Verification items for the finished model (mm, model axes). Round coordinates to 2 decimals unless told otherwise and drop trailing zeros. Write each loop counter-clockwise with the first axis right and the second up, starting at its lowest first coordinate (ties: lowest second). Pieces come first, ordered by that corner, then holes. Notation, with made-up numbers: M 47.25,28.5 L 78.25,28.5 A13 ccw 78.25,36.5 Z; hole C -5,89.25 d2. An arc over 180 degrees is marked long. One line per item, written item: value. Start each with the question number.
Item 1: Section check A-A, the plane x = -90.5. Record the cut outline in (y, z) (3 decimals).
Item 2: Section check C-C, the plane x = -71. Record the cut outline in (y, z) (1 decimal).
Item 3: Thickness scan on probe 1 along X at (y, z) = (-37.5, 1.1); probe 2 along X at (y, z) = (-17, 0.45); probe 3 along Y at (x, z) = (-71.5, 3). Record the ranges inside material, lowest first. Write a range as from..to.
Item 4: Gauge pin test, flat end, axial feed: pin 1 (18.5 mm diameter, centred on x = -76.93, y = -28.23, fed in from -Z). Record the tip position at first contact, or that the pin passes through.
Item 5: Section check D-D, the plane y = -11.5. Record the cut outline in (x, z) (3 decimals), then the cut area to 3 significant figures.
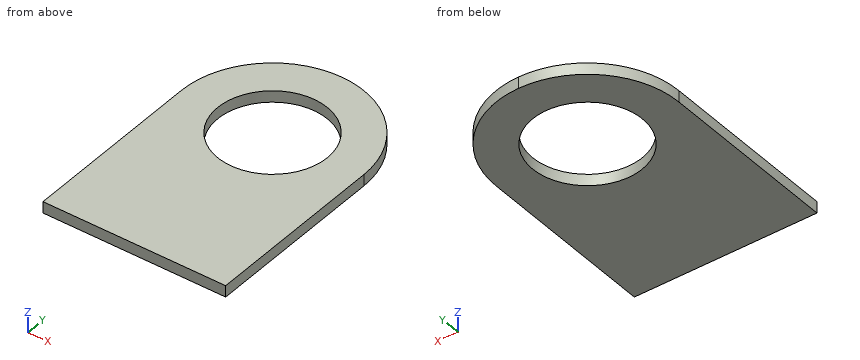
from build123d import *

# Parameters (mm, degrees)
SKETCH1_W           = 50.8
SKETCH1_H           = 76.2
SKETCH1_R           = 15.24
BOSS_EXTRUDE1_DEPTH = 3.175
FILLET1_R           = 25.4


with BuildPart() as part:
    # Sketch1 → Boss-Extrude1 (new body)
    with BuildSketch(Plane.XY):
        with Locations((-76.925714286, -40.930285714)):
            Rectangle(SKETCH1_W, SKETCH1_H)
        with Locations((-76.925714286, -28.230285714)):
            Circle(SKETCH1_R, mode=Mode.SUBTRACT)
    extrude(amount=BOSS_EXTRUDE1_DEPTH)

    # Fillet1
    fillet1_edges = [part.edges().sort_by_distance(p)[0] for p in [
        (-102.325714286, -2.830285714, 1.5875),
        (-51.525714286, -2.830285714, 1.5875),
    ]]
    fillet(fillet1_edges, radius=FILLET1_R - 0.0001)  # a hair under: the kernel refuses the full size


solid = part.part
Response values:
1. outline: M -79.03,0 L -35.158,0 L -35.158,3.175 L -79.03,3.175 Z; M -21.302,0 L -6.762,0 L -6.762,3.175 L -21.302,3.175 Z
2. outline: M -79,0 L -42.3,0 L -42.3,3.2 L -79,3.2 Z; M -14.2,0 L -3.5,0 L -3.5,3.2 L -14.2,3.2 Z
3. probe 1: x = -102.33..-89.02, -64.83..-51.53
3. probe 2: x = -99.71..-87.23, -66.62..-54.14
3. probe 3: y = -79.03..-42.47, -13.99..-3.42
4. pin 1: passes through
5. outline: M -96.037,0 L -57.814,0 L -57.814,3.175 L -96.037,3.175 Z
5. area: 121 mm2
